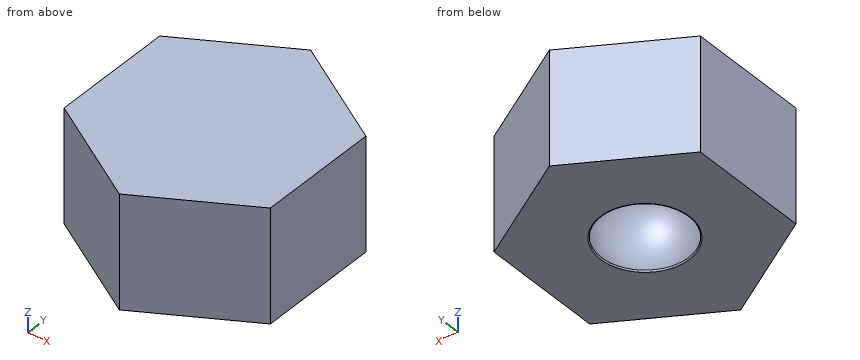
from build123d import *

# Parameters (mm, degrees)
BOSS_EXTRUDE1_DEPTH = 13.97


with BuildPart() as part:
    # Sketch1 → Boss-Extrude1 (new body)
    with BuildSketch(Plane.XY):
        Polygon((0, 14.664696837), (-12.7, 7.332348419), (-12.7, -7.332348419), (0, -14.664696837), (12.7, -7.332348419), (12.7, 7.332348419), align=None)
    extrude(amount=BOSS_EXTRUDE1_DEPTH)

    # Sketch4 → Cut-Revolve1 (revolve, cut)
    with BuildSketch(Plane(origin=(0, 0, 0), x_dir=(0, 0, -1), z_dir=(1, 0, 0))):
        with BuildLine():
            Line((0, 5.479886784), (0, 10.067284703))
            Line((0, 10.067284703), (2.770121515, 10.067284703))
            Line((2.770121515, 10.067284703), (2.770121515, 0))
            Line((2.770121515, 0), (-9.929878485, 0))
            ThreePointArc((-9.929878485, 0), (-6.647991818, 5.559602556), (-0.1947035, 5.372438024))
            ThreePointArc((-0.1947035, 5.372438024), (-0.065637733, 5.368694733), (0, 5.479886784))
        make_face()
    revolve(axis=Axis((0, 0, 9.929878485), (0, 0, -1)), mode=Mode.SUBTRACT)


solid = part.part
Could you check a few things on this model? Use its own coordinates, in mm. Round coordinates to 2 decimals unless told otherwise and drop trailing zeros. Write each loop counter-clockwise with the first axis right and the second up, starting at its lowest first coordinate (ties: lowest second). Pieces come first, ordered by that corner, then holes. Notation, with made-up numbers: (-37.5, 39.25) - (18.5, 39.25) arc R24 cw to (18.5, 78.25) - close; hole circle Ø11 at (89, 6). An arc over 180 degrees is marked (long way). Use a Markdown table: item, result.
Q1. Please list where these lines run through material, in increasing order: L1, parallel to Y at x = -0.5, z = 1.5; L2, parallel to X at y = -2.25, z = 4.5; L3, parallel to Y at x = 3, z = 7.
Output values:
| item | result |
|---|---|
| L1 | -14.38 to -5.98, 5.98 to 14.38 |
| L2 | -12.7 to -5.87, 5.87 to 12.7 |
| L3 | -12.93 to -4.43, 4.43 to 12.93 |
Q2. I want a section at D-D (z = 6.5). List the corners of the cut face in (x, y) for me.
Output values:
| item | result |
|---|---|
| outline | (-12.7, -7.33) - (0, -14.66) - (12.7, -7.33) - (12.7, 7.33) - (0, 14.66) - (-12.7, 7.33) - close; hole circle Ø11.28 at (0, 0) |
Q3. I want a section at A-A (z = 1). List the corners of the cut face in (x, y) for me.
Output values:
| item | result |
|---|---|
| outline | (-12.7, -7.33) - (0, -14.66) - (12.7, -7.33) - (12.7, 7.33) - (0, 14.66) - (-12.7, 7.33) - close; hole circle Ø11.6 at (0, 0) |
Q4. For pin 1 (8 mm diameter, centred on x = -3, z = 6, fed in from -Y); pin 2 (8 mm diameter, centred on x = 5.5, z = 5.5, fed in from -Y); pin 3 (4 mm diameter, centred on x = 7.5, z = 10, fed in from -Y); pin 4 (5 mm diameter, centred on x = -8, z = 3, fed in from +Y), each with a flat end and sliding along its axis, tell me the tip position at first contact or that it passes through.
Output values:
| item | result |
|---|---|
| pin 1 | y = -14.66 |
| pin 2 | y = -13.8 |
| pin 3 | y = -11.49 |
| pin 4 | y = 11.49 |
Q5. I want a section at B-B (z = 10.75). List the corners of the cut face in (x, y) for me.
Output values:
| item | result |
|---|---|
| outline | (-12.7, -7.33) - (0, -14.66) - (12.7, -7.33) - (12.7, 7.33) - (0, 14.66) - (-12.7, 7.33) - close |
Q6. I want a section at C-C (x = -9.25). List the corners of the cut face in (y, z) for me, plus the area to 3 significant figures.
Output values:
| item | result |
|---|---|
| outline | (-9.32, 0) - (9.32, 0) - (9.32, 13.97) - (-9.32, 13.97) - close |
| area | 261 mm2 |
